Geometry: final body of the model. Coordinates: model frame, mm. Face numbers are marked on the shaded views. Give positions to 0.01 mm unless a question says otherwise; leave off trailing zeros.
Q1. Line query: L1, parallel to Y at x = 0, z = 7.75; L2, parallel to X at y = -3.5, z = 15.5; L3, parallel to Y at x = 8, z = 6. Output: solid intervals per line, ascending.
Q2. Pin query (flat end, axial travel): pin 1 (5 mm diameter, centred on y = 19.5, z = 13.5, fed in from +X); pin 2 (6.5 mm diameter, centred on x = -12, y = 18, fed in from +Z); pin 3 (6 mm diameter, centred on x = 3.5, z = 11, fed in from -Y). Return the tip coordinate at first contact, or that it passes through.
Q3. Draft query along X for the marked faces 1, 2 and 3. Return one class per face: pulls with the +X half, pulls with the -X half, needs draft (parallel to the pull), parting line crosses it, or undercut.
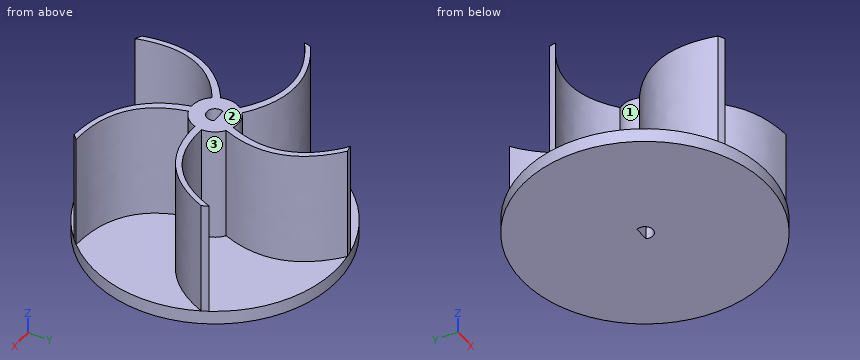
```python
from build123d import *

# Parameters (mm, degrees)
SKETCH1_R           = 26.5
SKETCH1_R_2         = 1.75
BOSS_EXTRUDE1_DEPTH = 3
SKETCH2_R           = 5
SKETCH2_R_2         = 1.75
BOSS_EXTRUDE2_DEPTH = 25
BOSS_EXTRUDE3_START = -28
BOSS_EXTRUDE3_DEPTH = 28
BOSS_EXTRUDE4_DEPTH = 25
CIRPATTERN1_COUNT   = 5


with BuildPart() as part:
    # Sketch1 → Boss-Extrude1 (new body)
    with BuildSketch(Plane.XY):
        Circle(SKETCH1_R)
        Circle(SKETCH1_R_2, mode=Mode.SUBTRACT)
    extrude(amount=BOSS_EXTRUDE1_DEPTH)

    # Sketch2 → Boss-Extrude2 (add)
    with BuildSketch(Plane.XY.offset(3)):
        Circle(SKETCH2_R)
        Circle(SKETCH2_R_2, mode=Mode.SUBTRACT)
    extrude(amount=BOSS_EXTRUDE2_DEPTH)

    # Sketch3 → Boss-Extrude3 (add)
    with BuildSketch(Plane.XY.offset(28).offset(BOSS_EXTRUDE3_START)):
        with BuildLine():
            ThreePointArc((1.58113883, 0.75), (0, 1.75), (-1.58113883, 0.75))
            Line((-1.58113883, 0.75), (0, 0.75))
            Line((0, 0.75), (1.58113883, 0.75))
        make_face()
    extrude(amount=BOSS_EXTRUDE3_DEPTH)

    # Sketch4 → Boss-Extrude4 (add)
    with BuildSketch(Plane.XY.offset(3)):
        with BuildLine():
            ThreePointArc((1.491525209, 4.772352937), (2.221644371, 4.479318731), (2.89676068, 4.075386799))
            add(Edge.make_bspline(
                [(2.89676068, 4.075386799), (6.200814746, 12.743614818), (4.154792704, 20.152161031), (-3.241305446, 26.301025436)],
                knots=[0.132924517, 0.132924517, 0.132924517, 0.132924517, 1, 1, 1, 1], degree=3))
            ThreePointArc((-3.241305446, 26.301025436), (-3.970865914, 26.200805787), (-4.697359939, 26.080352943))
            add(Edge.make_bspline(
                [(1.491525209, 4.772352937), (4.947392891, 13.120869253), (2.884431175, 20.223535921), (-4.697359939, 26.080352943)],
                knots=[0.156414662, 0.156414662, 0.156414662, 0.156414662, 1, 1, 1, 1], degree=3))
        make_face()
    boss_extrude4 = extrude(amount=BOSS_EXTRUDE4_DEPTH)

    # CirPattern1: Boss-Extrude4 ×5 about axis
    cirpattern1_axis = Axis((0, 0, 0), (0, 0, -1))
    for i in range(1, CIRPATTERN1_COUNT):
        add(boss_extrude4.rotate(cirpattern1_axis, i * 360 / CIRPATTERN1_COUNT))


solid = part.part
```
Data:
1. L1: y = -5 to -1.75, 0.75 to 5, 21.39 to 23.13
1. L2: x = -7.3 to -4.82, -3.57 to 3.57
1. L3: y = -16.45 to -15.05, -1.46 to 0.01
2. pin 1: stops at x = 3.57
2. pin 2: stops at z = 3
2. pin 3: stops at y = -15.41
3. face 1: pulls with the -X half
3. face 2: needs draft
3. face 3: undercut
